from build123d import *

# Parameters (mm, degrees)
BOSS_EXTRU_1_DEPTH      = 8
ESQUISSE2_R             = 17.5
ESQUISSE2_R_2           = 10
BOSS_EXTRU_2_DEPTH      = 15
ENL_V_START             = -10
ESQUISSE3_R             = 10
ENL_V_MAT_EXTRU_1_DEPTH = 10
ESQUISSE4_R             = 5
ENL_V_MAT_EXTRU_2_DEPTH = 10


with BuildPart() as part:
    # Esquisse1 → Boss.-Extru.1 (new body)
    with BuildSketch(Plane(origin=(0, 0, 0), x_dir=(1, 0, 0), z_dir=(0, 1, 0))):
        with BuildLine():
            Line((-15.074813432, 23), (-7, 45))
            Line((-7, 45), (7, 45))
            Line((7, 45), (15.074813432, 23))
            ThreePointArc((15.074813432, 23), (27.5, 0), (15.074813432, -23))
            Line((15.074813432, -23), (7, -45))
            Line((7, -45), (-7, -45))
            Line((-7, -45), (-15.074813432, -23))
            ThreePointArc((-15.074813432, -23), (-27.5, 0), (-15.074813432, 23))
        make_face()
    extrude(amount=BOSS_EXTRU_1_DEPTH)

    # Esquisse2 → Boss.-Extru.2 (add)
    with BuildSketch(Plane(origin=(0, 8, 0), x_dir=(1, 0, 0), z_dir=(0, 1, 0))):
        with Locations(Location((0, 0, 0), (0, 0, 90))):
            Circle(ESQUISSE2_R)
        with Locations(Location((0, 0, 0), (0, 0, 270))):
            Circle(ESQUISSE2_R_2, mode=Mode.SUBTRACT)
    extrude(amount=BOSS_EXTRU_2_DEPTH)

    # Esquisse3 → Enlèv. mat.-Extru.1 (cut)
    with BuildSketch(Plane(origin=(0, 8, 0), x_dir=(1, 0, 0), z_dir=(0, 1, 0)).offset(ENL_V_START)):
        with Locations(Location((0, 0, 0), (0, 0, 90))):
            Circle(ESQUISSE3_R)
    extrude(amount=ENL_V_MAT_EXTRU_1_DEPTH, mode=Mode.SUBTRACT)

    # Esquisse4 → Enlèv. mat.-Extru.2 (cut)
    with BuildSketch(Plane(origin=(0, 8, 0), x_dir=(1, 0, 0), z_dir=(0, 1, 0))):
        with Locations(Location((0, 35.5, 0), (0, 0, 270))):
            Circle(ESQUISSE4_R)
        with Locations(Location((0, -35.5, 0), (0, 0, 270))):
            Circle(ESQUISSE4_R)
    extrude(amount=-ENL_V_MAT_EXTRU_2_DEPTH, mode=Mode.SUBTRACT)


solid = part.part
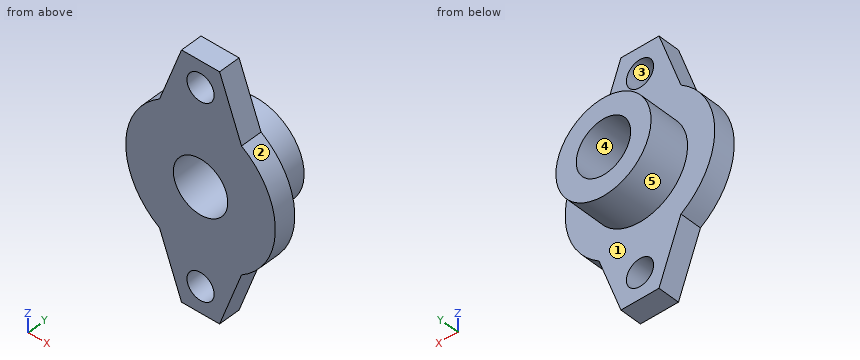
Input: part model. Units: mm. Frame: model coordinates. Face numbers are marked on the shaded views. A direction names the side the tool comes from. Round coordinates to 2 decimals unless told otherwise and drop trailing zeros. Order: outer loops, then holes, each group sorted by start corner. A loop starts at its lowest first (then second) coordinate and runs counter-clockwise, first axis right, second up. Notation, with made-up numbers: (36, 84.25) - (51, 84.25) arc R6 cw to (51, 90.25) - close; hole circle Ø5 at (-9.5, 50). An arc over 180 degrees is marked (long way). Answer as a JSON object with one key per item and string values. Group by question number.
(1) Cut plane A-A (x = 1). Return loops of the section in (y, z), then the cut area to 3 significant figures.
(2) Reachability of the marked faces 4 and 5 from +Z, -Z, +X, -X, +Y, -Y: full face, straight path, thin tool, end or side. Return the list, or none.
(3) Cut plane D-D (z = 0). Return loops of the section in (x, y).
(4) Draft query along X for the marked faces 1, 2 and 3. Return one class per face: released by +X, released by -X, zero draft, split by the parting line, or undercut.
(5) Pin query (flat end, axial travel): P1, Ø10, axis at x = -17, z = -14, coming from the -Y side; P2, Ø10, axis at x = 14.5, z = -21.5, coming from the +Y side; P3, Ø4, axis at x = 0.5, y = 16, coming from the +Z side. Return the tip coordinate at first contact, or that it passes through.
(6) Material intervals for probe 1 along X at (y, z) = (9, 0); probe 2 along Y at (x, z) = (-8, 39); probe 3 along X at (y, z) = (3, -0.5), sorted ascending. Write a range as from..to.
(7) Cut plane B-B (z = -35.5). Return loops of the section in (x, y).
(8) Cut plane C-C (y = 18). Return loops of the section in (x, z).
Here are the results:
{
 "1": {"outline": "(0, -45) - (8, -45) - (8, -40.4) - (0, -40.4) - close; (0, -30.6) - (8, -30.6) - (8, -17.47) - (23, -17.47) - (23, -9.95) - (0, -9.95) - close; (0, 9.95) - (23, 9.95) - (23, 17.47) - (8, 17.47) - (8, 30.6) - (0, 30.6) - close; (0, 40.4) - (8, 40.4) - (8, 45) - (0, 45) - close", "area": "630 mm^2"},
 "2": {"face 4": "+Y, -Y", "face 5": "+Y"},
 "3": {"outline": "(-27.5, 0) - (-10, 0) - (-10, 23) - (-17.5, 23) - (-17.5, 8) - (-27.5, 8) - close; (10, 0) - (27.5, 0) - (27.5, 8) - (17.5, 8) - (17.5, 23) - (10, 23) - close"},
 "4": {"face 1": "zero draft", "face 2": "released by +X", "face 3": "undercut"},
 "5": {"P1": "stops at y = 0", "P2": "stops at y = 8", "P3": "stops at z = 17.5"},
 "6": {"probe 1": "x = -17.5..-10, 10..17.5", "probe 2": "y = 0..8", "probe 3": "x = -27.5..-9.99, 9.99..27.5"},
 "7": {"outline": "(-10.49, 0) - (-5, 0) - (-5, 8) - (-10.49, 8) - close; (5, 0) - (10.49, 0) - (10.49, 8) - (5, 8) - close"},
 "8": {"outline": "circle Ø35 at (0, 0); hole circle Ø20 at (0, 0)"}
}
